from build123d import *

# Parameters (mm, degrees)
F0_W     = 42
F0_H     = 22
F0_R     = 2.25
F0_W_2   = 6
F0_H_2   = 2
F1_DEPTH = 25
F2_W     = 12
F2_H     = 6.5
F2_W_2   = 20
F2_W_3   = 30
F2_H_2   = 19
F3_DEPTH = 22
F4_DEPTH = 55
F5_DEPTH = 34
F6_DEPTH = 27


with BuildPart() as f1:
    # F0 (on Top) → F1 (new body)
    with BuildSketch(Plane.XY):
        with BuildLine():
            Line((44, 30), (-44, 30))
            Line((-44, 30), (-44, -30))
            Line((-44, -30), (6, -30))
            ThreePointArc((6, -30), (7.965431, -29.886003), (9.930862, -30))
            Line((9.930862, -30), (44, -30))
            Line((44, -30), (44, 0))
            Line((44, 0), (44, 30))
        make_face()
        with Locations((-19, -15)):
            Rectangle(F0_W, F0_H, mode=Mode.SUBTRACT)
        with Locations((-22.372717, 0)):
            Circle(F0_R, mode=Mode.SUBTRACT)
        with Locations((-29, 23)):
            Rectangle(F0_W_2, F0_H_2, mode=Mode.SUBTRACT)
        with Locations((-14, 23)):
            Rectangle(F0_W_2, F0_H_2, mode=Mode.SUBTRACT)
        with Locations((1, 23)):
            Rectangle(F0_W_2, F0_H_2, mode=Mode.SUBTRACT)
        with Locations((16, 23)):
            Rectangle(F0_W_2, F0_H_2, mode=Mode.SUBTRACT)
        with Locations((31, 23)):
            Rectangle(F0_W_2, F0_H_2, mode=Mode.SUBTRACT)
        with BuildLine():
            add(Edge.make_bspline(
                [(44, 0), (51.823881, -18.846294), (91.528348, -66.164455), (96, -85)],
                knots=[0, 0, 0, 0, 99.644368, 99.644368, 99.644368, 99.644368], degree=3))
            Line((44, 0), (44, -30))
            Line((44, -30), (9.930862, -30))
            ThreePointArc((9.930862, -30), (20.465431, -35.364284), (24.955334, -46.300163))
            Line((24.955334, -46.300163), (25.757433, -49.190948))
            ThreePointArc((25.757433, -49.190948), (40.09637, -57.581132), (40.434485, -74.190948))
            Line((40.434485, -74.190948), (41.236584, -77.081733))
            ThreePointArc((41.236584, -77.081733), (46.603334, -87.081733), (41.236584, -97.081733))
            Line((41.236584, -97.081733), (42.038683, -99.972518))
            Line((42.038683, -99.972518), (96, -85))
        make_face()
    extrude(amount=F1_DEPTH)

    # F2 (on face) → F3 (cut)
    with BuildSketch(Plane(origin=(0, 30, 0), x_dir=(-1, 0, 0), z_dir=(0, 1, 0))):
        with Locations((38, 12.5)):
            Rectangle(F2_W, F2_H)
        with Locations((22, 12.5)):
            Rectangle(F2_W_2, F2_H)
        Polygon((32, 22), (-11, 22), (-11, 3), (32, 3), (32, 9.25), (12, 9.25), (12, 15.75), (32, 15.75), align=None)
        with Locations((-26, 12.5)):
            Rectangle(F2_W_3, F2_H_2)
    extrude(amount=-F3_DEPTH, mode=Mode.SUBTRACT)

    # F2 (on face) → F4 (cut)
    with BuildSketch(Plane(origin=(0, 30, 0), x_dir=(-1, 0, 0), z_dir=(0, 1, 0))):
        with Locations((-26, 12.5)):
            Rectangle(F2_W_3, F2_H_2)
    extrude(amount=-F4_DEPTH, mode=Mode.SUBTRACT)

    # F2 (on face) → F5 (cut, through all)
    with BuildSketch(Plane(origin=(0, 30, 0), x_dir=(-1, 0, 0), z_dir=(0, 1, 0))):
        with Locations((22, 12.5)):
            Rectangle(F2_W_2, F2_H)
    extrude(amount=-F5_DEPTH, mode=Mode.SUBTRACT)

    # F2 (on face) → F6 (cut)
    with BuildSketch(Plane(origin=(0, 30, 0), x_dir=(-1, 0, 0), z_dir=(0, 1, 0))):
        with Locations((38, 12.5)):
            Rectangle(F2_W, F2_H)
    extrude(amount=-F6_DEPTH, mode=Mode.SUBTRACT)


solid = f1.part
Could you check a few things on this model? Use its own coordinates, in mm. A direction names the side the tool comes from. Give positions to 0.01 mm unless a question says otherwise; leave off trailing zeros. Order: outer loops, then holes, each group sorted by start corner. A loop starts at its lowest first (then second) coordinate and runs counter-clockwise, first axis right, second up.
1. I need wall thicknesses on L1, parallel to X at y = 0, z = 7.5; L2, parallel to X at y = 1, z = 12.5; L3, parallel to Y at x = -1.5, z = 6. Which ranges of each line are inside material? Lowest first, please.
2. We'd pull the mould along X, two halves only. Please class faces 4 (the flat face through (-6, 30, 2)), 5 (the flat face through (-44, 0, 12)), 6 (the flat face through (41, 3, 12)): pulls with the +X half, pulls with the -X half, needs draft (parallel to the pull), parting line crosses it, or undercut.
3. Suppose I cut it at C-C (y = -6). Give the number of separate pieces and of enclosed holes in the cut face, plus the area to 3 significant figures.
4. Suppose I cut it at A-A (x = -34.5). List the corners of the cut face in (y, z) for me, plus the area to 4 significant figures.
5. Suppose I cut it at B-B (x = 31). List the corners of the cut face in (y, z) for me.
6. For faces 1 (the flat face through (16, 22, 23)), 2 (the flat face through (40.83, -75.62, 12.32)), 3 (the flat face through (26, -25, 13)), which set-ups out of +Z, -Z, +X, -X, +Y, -Y let a thin tool reach every point of the face, with its end or its side?
7. Will these pins go through, and if not, where does the flat tip stop? P1, Ø2, axis at y = -29.5, z = 20.5, coming from the +X side; P2, Ø1.5, axis at x = -29, z = 1, coming from the -Y side; P3, Ø4.5, axis at y = 14, z = 18.5, coming from the +X side.
Solved:
1. L1: x = -44 to -24.62, -20.12 to 11, 41 to 44
1. L2: x = -44 to -32, -12 to 11, 41 to 44
1. L3: y = -30 to -26, -4 to 8
2. face 4: needs draft
2. face 5: pulls with the -X half
2. face 6: undercut
3. separate pieces: 2
3. enclosed holes: 1
3. area: 655 mm2
4. outline: (-30, 0) - (-26, 0) - (-26, 25) - (-30, 25) - close; (-4, 0) - (30, 0) - (30, 9.25) - (3, 9.25) - (3, 15.75) - (30, 15.75) - (30, 25) - (-4, 25) - close
4. area: 774.5 mm2
5. outline: (-50.12, 0) - (22, 0) - (22, 3) - (-25, 3) - (-25, 22) - (22, 22) - (22, 25) - (-50.12, 25) - close; (24, 0) - (30, 0) - (30, 3) - (24, 3) - close; (24, 22) - (30, 22) - (30, 25) - (24, 25) - close
6. face 1: +Z, -Z
6. face 2: +Z, -Z, -X, -Y
6. face 3: +Y
7. P1: stops at x = 62.91
7. P2: stops at y = -30
7. P3: stops at x = 44
